```python
from build123d import *

# Parameters (mm, degrees)
F3_R     = 60.074496
F4_DEPTH = 139


with BuildPart() as f1:
    # F0 (on Front) → F1 (revolve)
    with BuildSketch(Plane.XZ):
        Polygon((0, -31.509954), (0, 0), (-70.13493, 0), (-70.13493, -14.729742), (-74.609652, -19.950252), (-80.203056, -19.950252), (-88.033818, -26.289443), (-88.033818, -31.509954), align=None)
    revolve(axis=Axis((0, 0, -15.754977), (0, 0, -1)))

    # F2: F1 across face


with BuildPart() as f1_1:
    add(f1.part)
    add(f1.part.mirror(Plane.XY))

    # F3 (on face) → F4 (cut)
    with BuildSketch(Plane.XY.offset(31.509954)):
        Circle(F3_R)
    extrude(amount=-F4_DEPTH, mode=Mode.SUBTRACT)


solid = f1_1.part
```
Can you work these out from the model? Positions are in its coordinate system, mm. A direction names the side the tool comes from. Coordinates: 2 decimals unless noted, no trailing zeros. Loops run counter-clockwise (first coordinate to the right, second up) from the corner with the lowest first, then second, coordinate; pieces in that order, holes last. Notation, with made-up numbers: (-9, 12.5) -> (42, 12.5) arc R19 ccw to (42, 35.5) -> close; hole circle Ø2 at (26.5, 30.25). An arc over 180 degrees is marked (long way). Put each result on its own line as item: value. Start each with the question number.
Q1. For faces 1 (the face through (53, -53, 19.95)), 2 (the face through (-83.97, 26.44, 28.94)), which set-ups out of +Z, -Z, +X, -X, +Y, -Y let a thin tool reach every point of the face, with its end or its side?
Q2. I want a section at A-A (y = 0). Write out the boundary of the cut face in (x, z), plus the area to 3 significant figures.
Q3. If I drill on line 1 (Y direction, x = 0, z = 10.5); line 2 (X direction, y = -13, z = 4); line 3 (Z direction, x = 74, y = 35), over which ranges is the centre line in solid material (lowest first)? Write a range as [from, to].
Q4. I'm going to push flat-ended pins straight in: P1, Ø1, axis at y = 27.5, z = 8, coming from the +X side; P2, Ø8, axis at y = -60, z = 3, coming from the +X side; P3, Ø6, axis at x = 1.5, z = 5.5, coming from the +Y side. Where does each tip first touch, or does it pass through?
Q5. Thinking about a two-plate mould opening in Z: for faces 3 (the face through (-83.97, 26.44, -28.94)), 4 (the face through (53, -53, -19.95)), 5 (the face through (15.2, -68.47, 0.21)), 6 (the face through (-18.3, -57.5, -31.51)), which applies, pulls with the +Z half, pulls with the -Z half, needs draft (parallel to the pull), parting line crosses it, or undercut?
Q6. I want a section at C-C (z = 10.5). Write out the boundary of the cut face in (x, y).
Taken from the geometry:
1. face 1: none
1. face 2: +Z, -Z
2. outline: (-88.03, -31.51) -> (-60.07, -31.51) -> (-60.07, 31.51) -> (-88.03, 31.51) -> (-88.03, 26.29) -> (-80.2, 19.95) -> (-74.61, 19.95) -> (-70.13, 14.73) -> (-70.13, -14.73) -> (-74.61, -19.95) -> (-80.2, -19.95) -> (-88.03, -26.29) -> close; (60.07, -31.51) -> (88.03, -31.51) -> (88.03, -26.29) -> (80.2, -19.95) -> (74.61, -19.95) -> (70.13, -14.73) -> (70.13, 14.73) -> (74.61, 19.95) -> (80.2, 19.95) -> (88.03, 26.29) -> (88.03, 31.51) -> (60.07, 31.51) -> close
2. area: 2,040 mm2
3. line 1: y = [-70.13, -60.07], [60.07, 70.13]
3. line 2: x = [-68.92, -58.65], [58.65, 68.92]
3. line 3: z = [-31.51, -21.29], [21.29, 31.51]
4. P1: stops at x = 64.73
4. P2: stops at x = 42.22
4. P3: stops at y = 70.13
5. face 3: needs draft
5. face 4: undercut
5. face 5: undercut
5. face 6: pulls with the -Z half
6. outline: circle Ø140.27 at (0, 0); hole circle Ø120.15 at (0, 0)
